Could you check a few things on this drawing? It's one solid part, dimensions in mm from its lowest x, y, z. A direction names the side the tool comes from. Coordinates: 2 decimals unless noted, no trailing zeros. Write each loop counter-clockwise with the first axis right and the second up, starting at its lowest first coordinate (ties: lowest second). Pieces come first, ordered by that corner, then holes.
Item 1: I want a section at D-D (z = 14.25). Please give me the cut outline in (x, y).
Item 2: I want a section at B-B (z = 7.5). Please give me the cut outline in (x, y) (1 decimal).
Item 3: If we mould it in two halves opening along Z, with no side actions, what happens to the marked faces 1, 2 and 3? For each: pulls with the +Z half, pulls with the -Z half, needs draft (parallel to the pull), parting line crosses it, or undercut.
Item 4: I'm going to push flat-ended pins straight in: P1, Ø1.5, axis at x = 7.5, y = 2, coming from the +Z side; P2, Ø2, axis at x = 2.5, y = 1, coming from the -Z side (1 decimal). Where does each tip first touch, or does it pass through?
Item 5: I want a section at C-C (y = 2.9). Please give me the cut outline in (x, z), and give its area (3 significant figures).
Item 6: For the marked faces 4 and 5, which set-ups out of +Z, -Z, +X, -X, +Y, -Y let a thin tool reach every point of the face, with its end or its side?
Item 7: Please list where these lines run through material, in increasing order: line 1 (Y direction, x = 11.75, z = 14.75); line 2 (Z direction, x = 8.5, y = 2.6).
Item 8: I want a section at A-A (x = 8.5). Please give me the cut outline in (y, z).
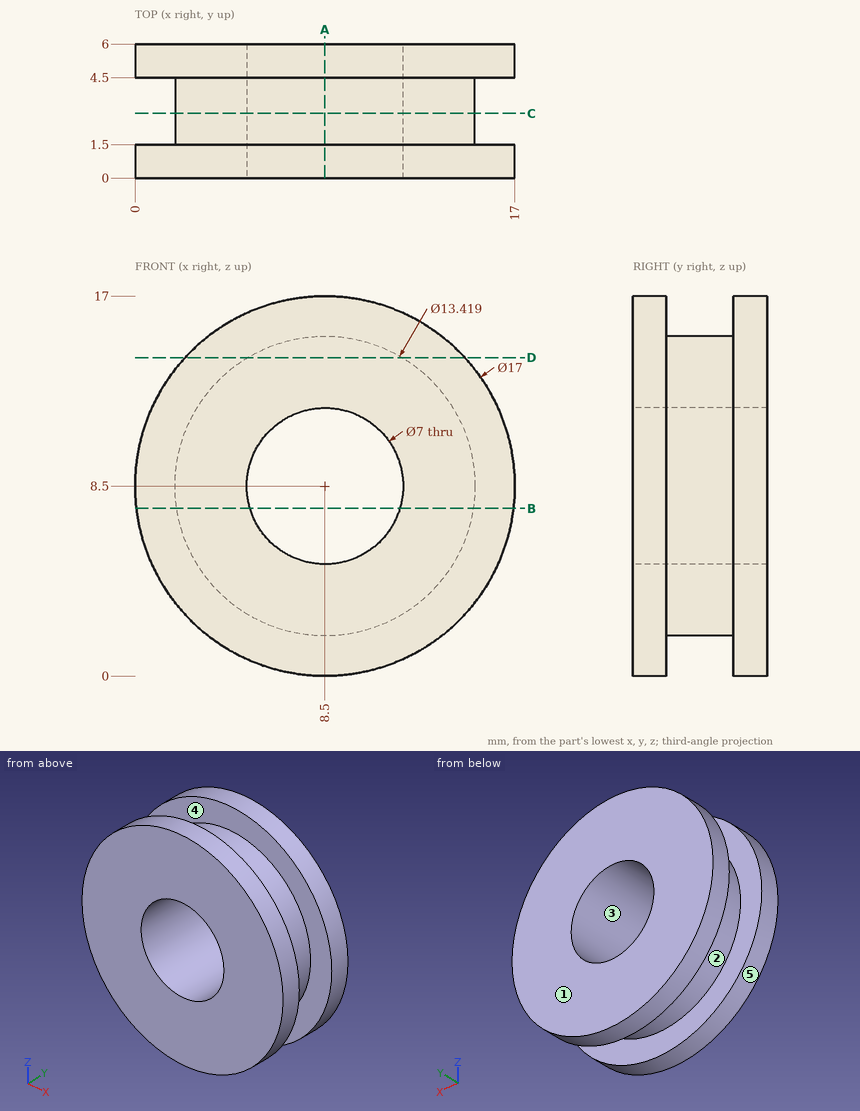
Answer:
1. outline: (2.24, 0) - (14.76, 0) - (14.76, 1.5) - (11.96, 1.5) - (11.96, 4.5) - (14.76, 4.5) - (14.76, 6) - (2.24, 6) - (2.24, 4.5) - (5.04, 4.5) - (5.04, 1.5) - (2.24, 1.5) - close
2. outline: (0.1, 0) - (5.1, 0) - (5.1, 6) - (0.1, 6) - (0.1, 4.5) - (1.9, 4.5) - (1.9, 1.5) - (0.1, 1.5) - close; (11.9, 0) - (16.9, 0) - (16.9, 1.5) - (15.1, 1.5) - (15.1, 4.5) - (16.9, 4.5) - (16.9, 6) - (11.9, 6) - close
3. face 1: needs draft
3. face 2: parting line crosses it
3. face 3: undercut
4. P1: stops at z = 16.99
4. P2: stops at z = 1.6
5. outline: circle Ø13.42 at (8.5, 8.5); hole circle Ø7 at (8.5, 8.5)
5. area: 103 mm2
6. face 4: none
6. face 5: +Y, -Y
7. line 1: y = 0 to 1.5, 4.5 to 6
7. line 2: z = 1.79 to 5, 12 to 15.21
8. outline: (0, 0) - (1.5, 0) - (1.5, 1.79) - (4.5, 1.79) - (4.5, 0) - (6, 0) - (6, 5) - (0, 5) - close; (0, 12) - (6, 12) - (6, 17) - (4.5, 17) - (4.5, 15.21) - (1.5, 15.21) - (1.5, 17) - (0, 17) - close
